from build123d import *

# Parameters (mm, degrees)
SKETCH_1_R      = 60
SKETCH_1_R_2    = 1.55
SKETCH_1_R_3    = 2.1
SKETCH_1_R_4    = 6
EXTRUDE_1_DEPTH = 3


with BuildPart() as part:
    # 草图1 → 凸台-拉伸1 (new body)
    with BuildSketch(Plane.XY):
        Circle(SKETCH_1_R)
        with Locations((0, 54.5)):
            Circle(SKETCH_1_R_2, mode=Mode.SUBTRACT)
        with Locations((-54.5, 0)):
            Circle(SKETCH_1_R_2, mode=Mode.SUBTRACT)
        with Locations((0, -54.5)):
            Circle(SKETCH_1_R_2, mode=Mode.SUBTRACT)
        with Locations((54.5, 0)):
            Circle(SKETCH_1_R_2, mode=Mode.SUBTRACT)
        with Locations((14.142135624, 14.142135624)):
            Circle(SKETCH_1_R_3, mode=Mode.SUBTRACT)
        with Locations((5.176380902, -19.318516526)):
            Circle(SKETCH_1_R_3, mode=Mode.SUBTRACT)
        with Locations((-19.318516526, 5.176380902)):
            Circle(SKETCH_1_R_3, mode=Mode.SUBTRACT)
        Circle(SKETCH_1_R_4, mode=Mode.SUBTRACT)
        with BuildLine():
            Line((3.923217687, -28.453617749), (6.022703538, -43.680396542))
            ThreePointArc((6.022703538, -43.680396542), (8.67451724, -47.877141015), (13.579927123, -48.639855873))
            ThreePointArc((13.579927123, -48.639855873), (35.70889245, -35.70889245), (48.639855873, -13.579927123))
            ThreePointArc((48.639855873, -13.579927123), (47.877141015, -8.67451724), (43.680396542, -6.022703538))
            Line((43.680396542, -6.022703538), (28.453617749, -3.923217687))
            ThreePointArc((28.453617749, -3.923217687), (25.717860997, -4.538114468), (24.057984584, -6.7980422))
            ThreePointArc((24.057984584, -6.7980422), (17.67766953, -17.67766953), (6.7980422, -24.057984584))
            ThreePointArc((6.7980422, -24.057984584), (4.538114468, -25.717860997), (3.923217687, -28.453617749))
        make_face(mode=Mode.SUBTRACT)
        with BuildLine():
            Line((28.453617749, 3.923217687), (43.680396542, 6.022703538))
            ThreePointArc((43.680396542, 6.022703538), (47.877141015, 8.67451724), (48.639855873, 13.579927123))
            ThreePointArc((48.639855873, 13.579927123), (35.70889245, 35.70889245), (13.579927123, 48.639855873))
            ThreePointArc((13.579927123, 48.639855873), (8.67451724, 47.877141015), (6.022703538, 43.680396542))
            Line((6.022703538, 43.680396542), (3.923217687, 28.453617749))
            ThreePointArc((3.923217687, 28.453617749), (4.538114468, 25.717860997), (6.7980422, 24.057984584))
            ThreePointArc((6.7980422, 24.057984584), (17.67766953, 17.67766953), (24.057984584, 6.7980422))
            ThreePointArc((24.057984584, 6.7980422), (25.717860997, 4.538114468), (28.453617749, 3.923217687))
        make_face(mode=Mode.SUBTRACT)
        with BuildLine():
            Line((-28.453617749, -3.923217687), (-43.680396542, -6.022703538))
            ThreePointArc((-43.680396542, -6.022703538), (-47.877141015, -8.67451724), (-48.639855873, -13.579927123))
            ThreePointArc((-48.639855873, -13.579927123), (-35.70889245, -35.70889245), (-13.579927123, -48.639855873))
            ThreePointArc((-13.579927123, -48.639855873), (-8.67451724, -47.877141015), (-6.022703538, -43.680396542))
            Line((-6.022703538, -43.680396542), (-3.923217687, -28.453617749))
            ThreePointArc((-3.923217687, -28.453617749), (-4.538114468, -25.717860997), (-6.7980422, -24.057984584))
            ThreePointArc((-6.7980422, -24.057984584), (-17.67766953, -17.67766953), (-24.057984584, -6.7980422))
            ThreePointArc((-24.057984584, -6.7980422), (-25.717860997, -4.538114468), (-28.453617749, -3.923217687))
        make_face(mode=Mode.SUBTRACT)
        with BuildLine():
            Line((-3.923217687, 28.453617749), (-6.022703538, 43.680396542))
            ThreePointArc((-6.022703538, 43.680396542), (-8.67451724, 47.877141015), (-13.579927123, 48.639855873))
            ThreePointArc((-13.579927123, 48.639855873), (-35.70889245, 35.70889245), (-48.639855873, 13.579927123))
            ThreePointArc((-48.639855873, 13.579927123), (-47.877141015, 8.67451724), (-43.680396542, 6.022703538))
            Line((-43.680396542, 6.022703538), (-28.453617749, 3.923217687))
            ThreePointArc((-28.453617749, 3.923217687), (-25.717860997, 4.538114468), (-24.057984584, 6.7980422))
            ThreePointArc((-24.057984584, 6.7980422), (-17.67766953, 17.67766953), (-6.7980422, 24.057984584))
            ThreePointArc((-6.7980422, 24.057984584), (-4.538114468, 25.717860997), (-3.923217687, 28.453617749))
        make_face(mode=Mode.SUBTRACT)
    extrude(amount=EXTRUDE_1_DEPTH)


solid = part.part
Verification items for the finished model (mm, model axes). Round coordinates to 2 decimals unless told otherwise and drop trailing zeros. Order: outer loops, then holes, each group sorted by start corner. A loop starts at its lowest first (then second) coordinate and runs counter-clockwise, first axis right, second up.
1. Release check for a two-part mould opening along Y. For faces 1 (the flat face through (-1, -12, 3)), 2 (the cylindrical face through (-17.551, -17.803, 1.479)) record: +Y half, -Y half, draft (parallel to the pull), parting line (faces both ways), or undercut.
Final values:
face 1: draft
face 2: undercut
2. Section check A-A on x = -40.5. Record the cut outline in (y, z), then the cut area to 3 significant figures.
Final values:
outline: (-44.27, 0) - (-30.17, 0) - (-30.17, 3) - (-44.27, 3) - close; (-5.58, 0) - (5.58, 0) - (5.58, 3) - (-5.58, 3) - close; (30.17, 0) - (44.27, 0) - (44.27, 3) - (30.17, 3) - close
area: 118 mm2
3. Section check B-B on y = -54.5. Record the cut outline in (x, z).
Final values:
outline: (-25.09, 0) - (-1.55, 0) - (-1.55, 3) - (-25.09, 3) - close; (1.55, 0) - (25.09, 0) - (25.09, 3) - (1.55, 3) - close
4. Thickness scan on L1, parallel to Y at x = 0, z = 1.5; L2, parallel to X at y = -27, z = 2; L3, parallel to Y at x = 34, z = 1.45. Record the ranges inside material, lowest first.
Final values:
L1: y = -60 to -56.05, -52.95 to -6, 6 to 52.95, 56.05 to 60
L2: x = -53.58 to -42.68, -3.99 to 3.99, 42.68 to 53.58
L3: y = -49.44 to -37.34, -4.69 to 4.69, 37.34 to 49.44
5. Go/stop test with flat-tipped pins: P1, Ø1, axis at y = -6.5, z = 0.5, coming from the -X side; P2, Ø1.5, axis at y = 11.5, z = 2, coming from the -X side; P3, Ø1, axis at x = -0.5, z = 2, coming from the -Y side. Record where each tip stops, or that it passes through.
Final values:
P1: stops at x = -59.7
P2: stops at x = -59.03
P3: stops at y = -60
6. Section check D-D on y = 39.5. Record the cut outline in (x, z), then the cut area to 3 significant figures.
Final values:
outline: (-45.16, 0) - (-31.46, 0) - (-31.46, 3) - (-45.16, 3) - close; (-5.45, 0) - (5.45, 0) - (5.45, 3) - (-5.45, 3) - close; (31.46, 0) - (45.16, 0) - (45.16, 3) - (31.46, 3) - close
area: 115 mm2
